```python
from build123d import *

# Parameters (mm, degrees)
F0_R     = 0.05
F0_R_2   = 10.31875
F0_R_3   = 2
F1_DEPTH = 10
F2_R     = 127


with BuildPart() as f1:
    # F0 (on Front) → F1 (new body)
    with BuildSketch(Plane.XZ):
        Polygon((508, 358.775), (508, 508), (358.775, 508), (358.775, 482.6), (263.525, 482.6), (263.525, 508), (203.2, 508), (203.2, 482.6), (107.95, 482.6), (107.95, 508), (47.625, 508), (47.625, 482.6), (-47.625, 482.6), (-47.625, 508), (-107.95, 508), (-107.95, 482.6), (-203.2, 482.6), (-203.2, 508), (-263.525, 508), (-263.525, 482.6), (-358.775, 482.6), (-358.775, 508), (-508, 508), (-508, 358.775), (-482.6, 358.775), (-482.6, 263.525), (-508, 263.525), (-508, 203.2), (-482.6, 203.2), (-482.6, 107.95), (-508, 107.95), (-508, 47.625), (-482.6, 47.625), (-482.6, -47.625), (-508, -47.625), (-508, -107.95), (-482.6, -107.95), (-482.6, -203.2), (-508, -203.2), (-508, -263.525), (-482.6, -263.525), (-482.6, -358.775), (-508, -358.775), (-508, -508), (-358.775, -508), (-358.775, -482.6), (-263.525, -482.6), (-263.525, -508), (-203.2, -508), (-203.2, -482.6), (-107.95, -482.6), (-107.95, -508), (-47.625, -508), (-47.625, -482.6), (47.625, -482.6), (47.625, -508), (107.95, -508), (107.95, -482.6), (203.2, -482.6), (203.2, -508), (263.525, -508), (263.525, -482.6), (358.775, -482.6), (358.775, -508), (508, -508), (508, -358.775), (482.6, -358.775), (482.6, -263.525), (508, -263.525), (508, -203.2), (482.6, -203.2), (482.6, -107.95), (508, -107.95), (508, -47.625), (482.6, -47.625), (482.6, 47.625), (508, 47.625), (508, 107.95), (482.6, 107.95), (482.6, 203.2), (508, 203.2), (508, 263.525), (482.6, 263.525), (482.6, 358.775), align=None)
        with Locations((-254, -381)):
            Circle(F0_R, mode=Mode.SUBTRACT)
        with Locations((-243.68125, -370.68125)):
            Circle(F0_R_2, mode=Mode.SUBTRACT)
        with Locations((-243.68125, -137.31875)):
            Circle(F0_R_2, mode=Mode.SUBTRACT)
        with Locations((-254, -127)):
            Circle(F0_R, mode=Mode.SUBTRACT)
        with Locations((-10.31875, -116.68125)):
            Circle(F0_R_2, mode=Mode.SUBTRACT)
        with BuildLine():
            ThreePointArc((0.0499998533, -380.9998788613), (0.0499999633, -380.9999394306), (0.05, -381))
            ThreePointArc((0.05, -381), (-6.05694e-05, -381.0499999633), (-0.0499998533, -380.9998788613))
            ThreePointArc((-0.0499998533, -380.9998788613), (-7.2787590143, -363.3671356466), (10.31875, -370.68125))
            ThreePointArc((10.31875, -370.68125), (7.3141143534, -377.9600090143), (0.0499998533, -380.9998788613))
        make_face(mode=Mode.SUBTRACT)
        with Locations((243.68125, -370.68125)):
            Circle(F0_R_2, mode=Mode.SUBTRACT)
        with Locations((254, -381)):
            Circle(F0_R, mode=Mode.SUBTRACT)
        with Locations((0, -127)):
            Circle(F0_R, mode=Mode.SUBTRACT)
        with BuildLine():
            ThreePointArc((253.9998788613, -126.9500001467), (254.0353124841, -126.9646018579), (254.05, -127))
            ThreePointArc((254.05, -127), (254.0353124841, -127.0353981421), (253.9998788613, -127.0499998533))
            ThreePointArc((253.9998788613, -127.0499998533), (233.3625, -127), (253.9998788613, -126.9500001467))
        make_face(mode=Mode.SUBTRACT)
        with Locations((-10.31875, 116.6792185501)):
            Circle(F0_R_2, mode=Mode.SUBTRACT)
        with Locations((-254, 127)):
            Circle(F0_R, mode=Mode.SUBTRACT)
        with Locations((-243.68125, 137.2707814499)):
            Circle(F0_R_2, mode=Mode.SUBTRACT)
        with Locations((-243.68125, 370.68125)):
            Circle(F0_R_2, mode=Mode.SUBTRACT)
        with Locations((-254, 381)):
            Circle(F0_R, mode=Mode.SUBTRACT)
        with Locations((0, 127)):
            Circle(F0_R, mode=Mode.SUBTRACT)
        with BuildLine():
            ThreePointArc((253.9998788613, 127.0499998533), (254.0353124841, 127.0353981421), (254.05, 127))
            ThreePointArc((254.05, 127), (254.0353124841, 126.9646018579), (253.9998788613, 126.9500001467))
            ThreePointArc((253.9998788613, 126.9500001467), (233.3625, 127), (253.9998788613, 127.0499998533))
        make_face(mode=Mode.SUBTRACT)
        with BuildLine():
            ThreePointArc((-0.0499998533, 380.9998788613), (-6.05694e-05, 381.0499999633), (0.05, 381))
            ThreePointArc((0.05, 381), (0.0499999633, 380.9999394306), (0.0499998533, 380.9998788613))
            ThreePointArc((0.0499998533, 380.9998788613), (7.3141143534, 377.9600090143), (10.31875, 370.68125))
            ThreePointArc((10.31875, 370.68125), (-7.2787590143, 363.3671356466), (-0.0499998533, 380.9998788613))
        make_face(mode=Mode.SUBTRACT)
        with Locations((243.68125, 370.68125)):
            Circle(F0_R_2, mode=Mode.SUBTRACT)
        with Locations((254, 381)):
            Circle(F0_R, mode=Mode.SUBTRACT)
        with Locations((-243.68125, 370.68125)):
            Circle(F0_R_2)
        with Locations((-243.68125, 370.68125)):
            Circle(F0_R_3, mode=Mode.SUBTRACT)
        with BuildLine():
            ThreePointArc((0.0499998533, 380.9998788613), (0, 380.95), (-0.0499998533, 380.9998788613))
            ThreePointArc((-0.0499998533, 380.9998788613), (-7.2787590143, 363.3671356466), (10.31875, 370.68125))
            ThreePointArc((10.31875, 370.68125), (7.3141143534, 377.9600090143), (0.0499998533, 380.9998788613))
        make_face()
        with Locations((0, 370.68125)):
            Circle(F0_R_3, mode=Mode.SUBTRACT)
        with Locations((243.68125, 370.68125)):
            Circle(F0_R_2)
        with Locations((243.68125, 370.68125)):
            Circle(F0_R_3, mode=Mode.SUBTRACT)
        with Locations((-243.68125, 137.2707814499)):
            Circle(F0_R_2)
        with Locations((-243.68125, 137.2707814499)):
            Circle(F0_R_3, mode=Mode.SUBTRACT)
        with Locations((-10.31875, 116.6792185501)):
            Circle(F0_R_2)
        with Locations((-10.31875, 116.6792185501)):
            Circle(F0_R_3, mode=Mode.SUBTRACT)
        with BuildLine():
            ThreePointArc((253.9998788613, 126.9500001467), (253.95, 127), (253.9998788613, 127.0499998533))
            ThreePointArc((253.9998788613, 127.0499998533), (233.3625, 127), (253.9998788613, 126.9500001467))
        make_face()
        with Locations((243.68125, 127)):
            Circle(F0_R_3, mode=Mode.SUBTRACT)
        with Locations((-243.68125, -137.31875)):
            Circle(F0_R_2)
        with Locations((-243.68125, -137.31875)):
            Circle(F0_R_3, mode=Mode.SUBTRACT)
        with Locations((-10.31875, -116.68125)):
            Circle(F0_R_2)
        with Locations((-10.31875, -116.68125)):
            Circle(F0_R_3, mode=Mode.SUBTRACT)
        with BuildLine():
            ThreePointArc((253.9998788613, -127.0499998533), (253.95, -127), (253.9998788613, -126.9500001467))
            ThreePointArc((253.9998788613, -126.9500001467), (233.3625, -127), (253.9998788613, -127.0499998533))
        make_face()
        with Locations((243.68125, -127)):
            Circle(F0_R_3, mode=Mode.SUBTRACT)
        with Locations((243.68125, -370.68125)):
            Circle(F0_R_2)
        with Locations((243.68125, -370.68125)):
            Circle(F0_R_3, mode=Mode.SUBTRACT)
        with BuildLine():
            ThreePointArc((-0.0499998533, -380.9998788613), (0, -380.95), (0.0499998533, -380.9998788613))
            ThreePointArc((0.0499998533, -380.9998788613), (7.3141143534, -377.9600090143), (10.31875, -370.68125))
            ThreePointArc((10.31875, -370.68125), (-7.2787590143, -363.3671356466), (-0.0499998533, -380.9998788613))
        make_face()
        with Locations((0, -370.68125)):
            Circle(F0_R_3, mode=Mode.SUBTRACT)
        with Locations((-243.68125, -370.68125)):
            Circle(F0_R_2)
        with Locations((-243.68125, -370.68125)):
            Circle(F0_R_3, mode=Mode.SUBTRACT)
    extrude(amount=F1_DEPTH)

    # F2
    f2_edges = [f1.edges().sort_by_distance(p)[0] for p in [
        (-508, -5, 508),
        (508, -5, 508),
        (508, -5, -508),
        (-508, -5, -508),
    ]]
    fillet(f2_edges, radius=F2_R)


solid = f1.part
```
Work out the finished part from the listing and answer in its coordinate system (mm). Coordinates: 2 decimals unless noted, no trailing zeros. Loops run counter-clockwise (first coordinate to the right, second up) from the corner with the lowest first, then second, coordinate; pieces in that order, holes last. Notation, with made-up numbers: (0.5, -32.75) - (45.5, -32.75) arc R29 cw to (45.5, -1.75) - close; hole circle Ø6 at (87.5, 6). An arc over 180 degrees is marked (long way). Use a Markdown table: item, result.
Item 1: Find section A-A, the plane x = -165. Determine the outline of the cut face in (y, z).
Evaluation:
| item | result |
|---|---|
| outline | (-10, -482.6) - (0, -482.6) - (0, 482.6) - (-10, 482.6) - close |
Item 2: Consider probe 1 along X at (y, z) = (-9, -384); probe 2 along Z at (x, y) = (-163, -8.5). Determine where each line is inside the solid, lowest interval first. Write a range as from..to.
Evaluation:
| item | result |
|---|---|
| probe 1 | x = -507.96..507.96 |
| probe 2 | z = -482.6..482.6 |
Item 3: Given pin 1 Ø3 at (x, y) = (294.5, -7.5) entering from +Z; pin 2 Ø4 at (y, z) = (-2, 196.5) entering from +X; pin 3 Ø1.5 at (x, z) = (43, 235.5) entering from +Y; pin 4 Ø3.5 at (x, z) = (0, 370.68) entering from +Y, each flat-ended and moving along its own axis, determine where each tip first touches the part or whether it passes through.
Evaluation:
| item | result |
|---|---|
| pin 1 | stops at z = 482.6 |
| pin 2 | stops at x = 482.6 |
| pin 3 | stops at y = 0 |
| pin 4 | passes through |
Item 4: Find section B-B, the plane z = -342.5. Determine the outline of the cut face in (x, y).
Evaluation:
| item | result |
|---|---|
| outline | (-482.6, -10) - (482.6, -10) - (482.6, 0) - (-482.6, 0) - close |
